Part model, mm, in its own coordinate system. Round coordinates to 2 decimals unless told otherwise and drop trailing zeros. Order: outer loops, then holes, each group sorted by start corner. A loop starts at its lowest first (then second) coordinate and runs counter-clockwise, first axis right, second up. Notation, with made-up numbers: M 87.25,61.25 L 135.25,61.25 A20 ccw 135.25,83.25 Z; hole C -1,59 d10. An arc over 180 degrees is marked long. One line per question, with ' | ' between items.
from build123d import *

# Parameters (mm, degrees)
F0_W     = 36
F0_H     = 20
F1_DEPTH = 2.8
F2_R     = 1.25
F3_DEPTH = 25
F4_R     = 1


with BuildPart() as f1:
    # F0 (on Top) → F1 (new body, symmetric)
    with BuildSketch(Plane.XY):
        Rectangle(F0_W, F0_H)
    extrude(amount=F1_DEPTH, both=True)

    # F2 (on face) → F3 (join)
    with BuildSketch(Plane(origin=(-18, 0, 0), x_dir=(0, -1, 0), z_dir=(-1, 0, 0))):
        with Locations((-3.5708139185, -0.681526144)):
            Circle(F2_R)
        with Locations((4.1246912515, -0.681526144)):
            Circle(F2_R)
    extrude(amount=F3_DEPTH)

    # F4
    f4_edges = [f1.edges().sort_by_distance(p)[0] for p in [
        (0, -10, 2.8),
        (0, -10, -2.8),
        (0, 10, 2.8),
        (0, 10, -2.8),
    ]]
    fillet(f4_edges, radius=F4_R)


solid = f1.part
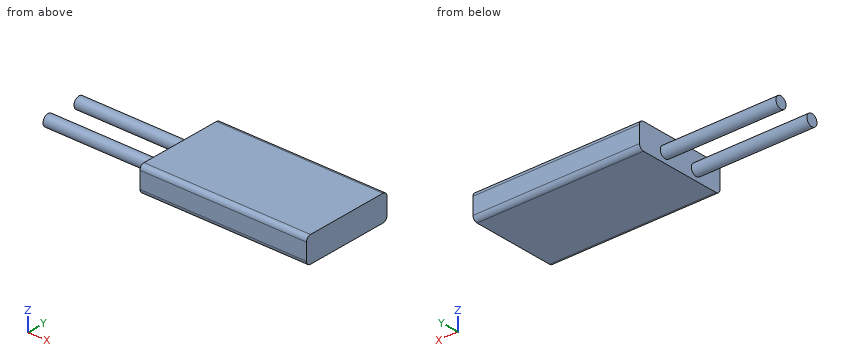
1) Saw through at A-A (y = 4). List the corners of the cut face in (x, z), plus the area to 3 significant figures.
The answers:
outline: M -43,-1.86 L -18,-1.86 L -18,-2.8 L 18,-2.8 L 18,2.8 L -18,2.8 L -18,0.49 L -43,0.49 Z | area: 260 mm²
2) Probe line 1 (Y direction, x = -32, z = -0.05); line 2 (X direction, y = -8.5, z = 0.8); line 3 (Y direction, x = -23, z = -1.6). List the from-to ranges inside material, lowest first. Write a range as [from, to].
The answers:
line 1: y = [-5.2, -3.05], [2.49, 4.65] | line 2: x = [-18, 18] | line 3: y = [-4.97, -3.28], [2.72, 4.42]
3) Saw through at C-C (x = -32.5). List the corners of the cut face in (y, z).
The answers:
outline: C -4.12,-0.68 d2.5; C 3.57,-0.68 d2.5
4) Saw through at D-D (y = -7.75). List the corners of the cut face in (x, z).
The answers:
outline: M -18,-2.8 L 18,-2.8 L 18,2.8 L -18,2.8 Z
5) Saw through at B-B (z = -0.1). List the corners of the cut face in (x, y), plus the area to 3 significant figures.
The answers:
outline: M -43,-5.23 L -18,-5.23 L -18,-10 L 18,-10 L 18,10 L -18,10 L -18,4.68 L -43,4.68 L -43,2.46 L -18,2.46 L -18,-3.02 L -43,-3.02 Z | area: 831 mm²
